Here's how the part is built. I have some questions about the finished solid (model axes, mm). A direction names the side the tool comes from. Give positions to 0.01 mm unless a question says otherwise; leave off trailing zeros. Write each loop counter-clockwise with the first axis right and the second up, starting at its lowest first coordinate (ties: lowest second). Pieces come first, ordered by that corner, then holes. Notation, with made-up numbers: (-5, 73.25) - (21, 73.25) arc R25 cw to (21, 109.25) - close; hole circle Ø1 at (-8, 60.25). An arc over 180 degrees is marked (long way). One line per item, written item: value. Start each with the question number.
1) I'm going to push flat-ended pins straight in: P1, Ø2, axis at y = -11, z = 3.5, coming from the -X side; P2, Ø2, axis at y = -11.5, z = 2, coming from the +X side; P3, Ø1, axis at y = -4.5, z = 1, coming from the +X side. Where does each tip first touch, or does it pass through?
2) On a 3-axis mill with a long thin cutter (end or side, diameter ignored), from which of +Z, -Z, +X, -X, +Y, -Y can I reach the whole of each face in a straight line? I mean faces 1 (the flat face through (0, -16, 2)), 2 (the flat face through (3, -3, 1.588)). Say none if no direction works.
3) Imagine slicing it at B-B on y = 1.75. Write out the boundary of the cut face in (x, z), plus the area to 3 significant figures.
4) Imagine slicing it at D-D on y = -14.25. Write out the boundary of the cut face in (x, z).
5) Imagine slicing it at C-C on x = 0.25. Write out the boundary of the cut face in (y, z), plus the area to 3 significant figures.
6) Imagine slicing it at A-A on z = 0.55. Write out the boundary of the cut face in (x, y).
7) Please list where these lines run through material, in increasing order: L1, parallel to X at y = -10.5, z = 1.8; L2, parallel to Z at x = -4, y = 2; L3, parallel to Y at x = -1.75, z = 2.05. Write a range as [from, to].
from build123d import *

# Parameters (mm, degrees)
F1_DEPTH = 1.5875
F2_W     = 2
F2_H     = 7
F3_DEPTH = 4


# Not quite as in the source:
# - ends of sketch curves that miss each other by under 0.0002 mm in the source are joined


with BuildPart() as f1:
    # F0 (on Top) → F1 (new body)
    with BuildSketch(Plane.XY):
        with BuildLine():
            Line((-3.52345, 0), (-6, 0))
            ThreePointArc((-6, 0), (-4.8989795096, -3.4641015812), (-2.0000000784, -5.6568542218))
            Line((-2.0000000784, -5.6568542218), (-2, -9))
            Line((-2, -9), (0, -9))
            Line((0, -9), (0, -3.52345))
            ThreePointArc((0, -3.52345), (-2.4914553882, -2.4914553882), (-3.52345, 0))
        make_face()
        with BuildLine():
            ThreePointArc((2.0000000784, -5.6568542218), (4.8989795096, -3.4641015812), (6, 0))
            Line((6, 0), (3.52345, 0))
            ThreePointArc((3.52345, 0), (2.4914553882, -2.4914553882), (0, -3.52345))
            Line((0, -3.52345), (0, -9))
            Line((0, -9), (2, -9))
            Line((2, -9), (2.0000000784, -5.6568542218))
        make_face()
        with BuildLine():
            ThreePointArc((6, 0), (4.2426406871, 4.2426406871), (0, 6))
            Line((0, 6), (0, 3.52345))
            ThreePointArc((0, 3.52345), (2.4914553882, 2.4914553882), (3.52345, 0))
            Line((3.52345, 0), (6, 0))
        make_face()
        with BuildLine():
            Line((0, 3.52345), (0, 6))
            ThreePointArc((0, 6), (-4.2426406871, 4.2426406871), (-6, 0))
            Line((-6, 0), (-3.52345, 0))
            ThreePointArc((-3.52345, 0), (-2.4914553882, 2.4914553882), (0, 3.52345))
        make_face()
    extrude(amount=F1_DEPTH)

    # F2 (on Top) → F3 (join)
    with BuildSketch(Plane.XY):
        with Locations((-1, -12.5)):
            Rectangle(F2_W, F2_H)
        with Locations((1, -12.5)):
            Rectangle(F2_W, F2_H)
    extrude(amount=F3_DEPTH)


solid = f1.part
Numbers:
1. P1: x = -2
1. P2: x = 2
1. P3: x = 4.47
2. face 1: +Z, -Z, +X, -X, -Y
2. face 2: +Z, +X, -X, +Y
3. outline: (-5.74, 0) - (-3.06, 0) - (-3.06, 1.59) - (-5.74, 1.59) - close; (3.06, 0) - (5.74, 0) - (5.74, 1.59) - (3.06, 1.59) - close
3. area: 8.51 mm^2
4. outline: (-2, 0) - (2, 0) - (2, 4) - (-2, 4) - close
5. outline: (-16, 0) - (-3.51, 0) - (-3.51, 1.59) - (-9, 1.59) - (-9, 4) - (-16, 4) - close; (3.51, 0) - (5.99, 0) - (5.99, 1.59) - (3.51, 1.59) - close
5. area: 40.6 mm^2
6. outline: (-2, -16) - (2, -16) - (2, -5.66) arc R6 ccw (long way) to (-2, -5.66) - close; hole circle Ø7.05 at (0, 0)
7. L1: [-2, 2]
7. L2: [0, 1.59]
7. L3: [-16, -9]
